Part model, mm, in its own coordinate system. A direction names the side the tool comes from. Give positions to 0.01 mm unless a question says otherwise; leave off trailing zeros. Loops run counter-clockwise (first coordinate to the right, second up) from the corner with the lowest first, then second, coordinate; pieces in that order, holes last. Notation, with made-up numbers: (-12.75, 60.25) -> (9.25, 60.25) arc R21 cw to (9.25, 91.25) -> close; hole circle Ø3 at (12.25, 82). An arc over 180 degrees is marked (long way). One line per question, with ' | ' between items.
Autodesk Inventor part; units mm, degrees
ref_plane "YZ Plane" through (0, 0, 0) normal (1, 0, 0) x (0, 1, 0)
ref_plane "XZ Plane" through (0, 0, 0) normal (0, 1, 0) x (-1, 0, 0)
ref_plane "XY Plane" through (0, 0, 0) normal (0, 0, 1) x (1, 0, 0)
sketch "Эскиз1" plane through (0, 0, 0) normal (0, 0, 1) x (1, 0, 0)
  circle A0 centre (0, 0) radius 2.75
extrude "Выдавливание1" add sketch "Эскиз1" along normal blind 15
sketch "Эскиз2" plane through (0, 0, 15) normal (0, 0, 1) x (1, 0, 0)
  circle A0 centre (0, 0) radius 2.75
  circle A1 centre (0, 0) radius 4
  dimension "d2" = 8
extrude "Выдавливание2" add sketch "Эскиз2" along normal blind 2 contours A0 | A1
sketch "Эскиз3" plane through (0, 0, 17) normal (0, 0, 1) x (1, 0, 0)
  circle A0 centre (0, 0) radius 2.75
  circle A1 centre (0, 0) radius 2
  dimension "d5" = 4
  dimension "d6" = 5.5
extrude "Выдавливание3" add sketch "Эскиз3" along normal blind 8 contours A1
sketch "Эскиз4" plane through (0, 0, 0) normal (0, 0, -1) x (-1, 0, 0)
  circle A0 centre (0, 0) radius 4
extrude "Выдавливание4" add sketch "Эскиз4" along normal blind 1
sketch "Эскиз5" plane through (0, 0, -1) normal (0, 0, -1) x (-1, 0, 0)
  circle A0 centre (0, 0) radius 4
  circle A1 centre (0, 0) radius 3
  dimension "d11" = 6
extrude "Выдавливание5" add sketch "Эскиз5" along normal blind 1
properties part number "butt"
1) Tool access for faces 4 (the flat face through (0, 0, -1)), 5 (the flat face through (-1, 3, -2)), 6 (the cylindrical face through (0, 2, 21)), 7 (the cylindrical face through (0.867, 3.905, -0.986)), 8 (the flat face through (3, 1, 15)): list every direction of +Z, -Z, +X, -X, +Y, -Y with a clear straight run to the whole face (end or side of a thin tool).
Found:
face 4: -Z | face 5: -Z, +X, -X, +Y, -Y | face 6: +Z | face 7: +Z, -Z | face 8: none
2) Saw through at D-D (y = 3.5). Give the cut face in (x, z), and give its area (3 significant figures).
Found:
outline: (-1.94, -2) -> (1.94, -2) -> (1.94, 0) -> (-1.94, 0) -> close; (-1.94, 15) -> (1.94, 15) -> (1.94, 17) -> (-1.94, 17) -> close | area: 15.5 mm2
3) Drill centre lines: line 1 (Y direction, x = 0, z = -1.2); line 2 (Z direction, x = 2.5, y = -3); line 3 (Z direction, x = 0.5, y = 2). Where is each one in solid material? Low to high.
Found:
line 1: -4 to -3, 3 to 4 | line 2: -2 to 0, 15 to 17 | line 3: -1 to 17
4) Saw through at C-C (z = 16.5). Give the cut face in (x, y), and give its area (3 significant figures).
Found:
outline: circle Ø8 at (0, 0) | area: 50.3 mm2
5) Pull direction Y, two halves, no side cores. Call faces 1 (the cylindrical face through (-0.596, 2.685, 7.395)), 2 (the cylindrical face through (3, -0.1, -1.5)), 3 (the flat face through (0, 0, 25)): pulls with the +Y half, pulls with the -Y half, needs draft (parallel to the pull), parting line crosses it, or undercut.
Found:
face 1: parting line crosses it | face 2: undercut | face 3: needs draft
6) Saw through at A-A (y = 0). Give the cut face in (x, z), and give its area (4 significant figures).
Found:
outline: (-4, -2) -> (-3, -2) -> (-3, -1) -> (3, -1) -> (3, -2) -> (4, -2) -> (4, 0) -> (2.75, 0) -> (2.75, 15) -> (4, 15) -> (4, 17) -> (2, 17) -> (2, 25) -> (-2, 25) -> (-2, 17) -> (-4, 17) -> (-4, 15) -> (-2.75, 15) -> (-2.75, 0) -> (-4, 0) -> close | area: 140.5 mm2
7) Pin check, flat tips, straight feed: P1, Ø3, axis at x = -1.5, z = 13, coming from the +Y side; P2, Ø1.5, axis at x = 2.5, z = 18, coming from the +Y side; P3, Ø1, axis at x = 1, z = 20, coming from the +Y side. Stop position of each tip, or through.
Found:
P1: y = 2.75 | P2: y = 0.97 | P3: y = 1.94
